from build123d import *

# Parameters (mm, degrees)
SKETCH1_W             = 100
SKETCH1_H             = 123
BOSS_EXTRUDE1_DEPTH   = 3
SKETCH2_R             = 4
BOSS_EXTRUDE2_DEPTH   = 5
CUT_EXTRUDE1_DEPTH    = 80.418196907
FILLET1_R             = 4
BOSS_EXTRUDE3_DEPTH   = 3
M4X0_7_TAPPED_HOLE1_D = 3.3


with BuildPart() as part:
    # Sketch1 → Boss-Extrude1 (new body)
    with BuildSketch(Plane(origin=(0, 0, 0), x_dir=(1, 0, 0), z_dir=(0, 1, 0))):
        Rectangle(SKETCH1_W, SKETCH1_H)
    extrude(amount=BOSS_EXTRUDE1_DEPTH)

    # Sketch2 → Boss-Extrude2 (add)
    with BuildSketch(Plane(origin=(0, 3, 0), x_dir=(1, 0, 0), z_dir=(0, 1, 0))):
        with Locations(Location((46, 57.5, 0), (0, 0, 90))):
            Circle(SKETCH2_R)
        with Locations(Location((46, -57.5, 0), (0, 0, 270))):
            Circle(SKETCH2_R)
        with Locations(Location((-46, -57.5, 0), (0, 0, 270))):
            Circle(SKETCH2_R)
        with Locations(Location((-46, 57.5, 0), (0, 0, 90))):
            Circle(SKETCH2_R)
    extrude(amount=BOSS_EXTRUDE2_DEPTH)

    # Sketch3 → Cut-Extrude1 (cut, through all)
    with BuildSketch(Plane(origin=(0, 3, 0), x_dir=(1, 0, 0), z_dir=(0, 1, 0))):
        with BuildLine():
            Line((-43, 46.916994756), (-43, -46.916994756))
            ThreePointArc((-43, -46.916994756), (-38.221825407, -49.721825407), (-35.416994756, -54.5))
            Line((-35.416994756, -54.5), (35.416994756, -54.5))
            ThreePointArc((35.416994756, -54.5), (38.221825407, -49.721825407), (43, -46.916994756))
            Line((43, -46.916994756), (43, 46.916994756))
            ThreePointArc((43, 46.916994756), (38.221825407, 49.721825407), (35.416994756, 54.5))
            Line((35.416994756, 54.5), (-35.416994756, 54.5))
            ThreePointArc((-35.416994756, 54.5), (-38.221825407, 49.721825407), (-43, 46.916994756))
        make_face()
    extrude(amount=-CUT_EXTRUDE1_DEPTH, mode=Mode.SUBTRACT)

    # Fillet1
    fillet1_edges = [part.edges().sort_by_distance(p)[0] for p in [
        (-50, 1.5, -61.5),
        (50, 1.5, -61.5),
        (50, 1.5, 61.5),
        (-50, 1.5, 61.5),
    ]]
    fillet(fillet1_edges, radius=FILLET1_R)

    # Sketch4 → Boss-Extrude3 (add, through all)
    with BuildSketch(Plane(origin=(0, 3, 0), x_dir=(1, 0, 0), z_dir=(0, 1, 0))):
        Polygon((-43.657393572, 59.374085143), (-48.342606428, 55.625914857), (-3.841874542, 0), (-48.342606428, -55.625914857), (-43.657393572, -59.374085143), (0, -4.802343178), (43.657393572, -59.374085143), (48.342606428, -55.625914857), (3.841874542, 0), (48.342606428, 55.625914857), (43.657393572, 59.374085143), (0, 4.802343178), align=None)
    extrude(amount=-BOSS_EXTRUDE3_DEPTH)

    # M4x0.7 Tapped Hole1 (through all)
    with Locations(Plane(origin=(0, 8, 0), x_dir=(1, 0, 0), z_dir=(0, 1, 0))):
        with Locations((-46, 57.5), (46, 57.5), (46, -57.5), (-46, -57.5)):
            Hole(M4X0_7_TAPPED_HOLE1_D / 2)


solid = part.part
Model file for the job. Use its own axes, mm. A direction names the side the tool comes from. Coordinates: 2 decimals unless noted, no trailing zeros. Write each loop counter-clockwise with the first axis right and the second up, starting at its lowest first coordinate (ties: lowest second). Pieces come first, ordered by that corner, then holes. Notation, with made-up numbers: (-17.5, 43) - (14.5, 43) arc R16 ccw to (14.5, 67) - close; hole circle Ø6 at (80.25, 74). An arc over 180 degrees is marked (long way). Write each question's results on one line, items separated by ' | '. Start each with the question number.
1) Cut at B-B (x = -7). Write the cut outline in (y, z).
2) 3-axis set-ups, long thin cutter, end or side, ignore diameter. For faces 1 (the face through (44.799, 5.465, -61.315)), 2 (the face through (-50, 1, 1)), 3 (the face through (-23.05, 1.52, -24.01)): which of +Z, -Z, +X, -X, +Y, -Y reach the whole face in a straight line?
3) Cut at A-A (y = 5). Write the cut outline in (x, z), then the cut area to 3 significant figures.
4) Probe line 1 along Z through (x, y) = (-46, 5.5); line 2 along Z through (x, y) = (-46, 2.75). List the from-to ranges inside material, lowest first. Write a range as from..to.
5) Mould opens along Z. For faces 4 (the face through (36.097, 1.521, -52.711)), 5 (the face through (-48, 8, 57)), 6 (the face through (48.797, 1.521, -60.359)) say: pulls with the +Z half, pulls with the -Z half, needs draft (parallel to the pull), parting line crosses it, or undercut.
6) Flat gauge pins, fed straight in: P1, Ø4.5, axis at x = -46, z = 57.5, coming from the -Y side; P2, Ø8, axis at x = -11.5, z = 21, coming from the +Y side. Where does each tip first touch, or does it go through?
7) Cut at C-C (z = -23.5). Write the cut outline in (x, y).
Returned:
1) outline: (0, -61.5) - (3, -61.5) - (3, -54.5) - (0, -54.5) - close; (0, -13.55) - (3, -13.55) - (3, -3.95) - (0, -3.95) - close; (0, 3.95) - (3, 3.95) - (3, 13.55) - (0, 13.55) - close; (0, 54.5) - (3, 54.5) - (3, 61.5) - (0, 61.5) - close
2) face 1: +Y | face 2: +Z, -Z, -X, +Y, -Y | face 3: +Y, -Y
3) outline: circle Ø8 at (-46, -57.5); circle Ø8 at (-46, 57.5); circle Ø8 at (46, -57.5); circle Ø8 at (46, 57.5); hole circle Ø3.3 at (-46, -57.5); hole circle Ø3.3 at (-46, 57.5); hole circle Ø3.3 at (46, -57.5); hole circle Ø3.3 at (46, 57.5) | area: 167 mm^2
4) line 1: -61.5..-59.15, -55.85..-53.5, 53.5..55.85, 59.15..61.5 | line 2: -61.5..-59.15, -55.85..55.85, 59.15..61.5
5) face 4: undercut | face 5: needs draft | face 6: pulls with the -Z half
6) P1: y = 0 | P2: y = 3
7) outline: (-50, 0) - (-43, 0) - (-43, 3) - (-50, 3) - close; (-22.64, 0) - (-14.96, 0) - (-14.96, 3) - (-22.64, 3) - close; (14.96, 0) - (22.64, 0) - (22.64, 3) - (14.96, 3) - close; (43, 0) - (50, 0) - (50, 3) - (43, 3) - close
